```python
from build123d import *

# Parameters (mm, degrees)
ESQUISSE1_W                                        = 50.5
ESQUISSE1_H                                        = 26.5
ESQUISSE1_R                                        = 1.1
BOSS_EXTRU_1_DEPTH                                 = 3
CONG_1_R                                           = 1
CHAMBRAGE_POUR_VIS_SIX_PANS_CREUX_M1_6_D           = 2.2
CHAMBRAGE_POUR_VIS_SIX_PANS_CREUX_M1_6_CBORE_D     = 3.8
CHAMBRAGE_POUR_VIS_SIX_PANS_CREUX_M1_6_CBORE_DEPTH = 1.2
BOSS_EXTRU_2_START                                 = -19
ESQUISSE4_R                                        = 1.6
ESQUISSE4_W                                        = 11.6
ESQUISSE4_H                                        = 26.5
BOSS_EXTRU_2_DEPTH                                 = 19
ENL_V_START                                        = -19
ENL_V_MAT_EXTRU_1_DEPTH                            = 7
ESQUISSE6_W                                        = 11.6
ESQUISSE6_H                                        = 6
ENL_V_MAT_EXTRU_2_DEPTH                            = 50.487191272
BOSS_EXTRU_3_DEPTH                                 = 2
CHANFREIN1_SIZE                                    = 1


with BuildPart() as part:
    # Esquisse1 → Boss.-Extru.1 (new body)
    with BuildSketch(Plane(origin=(0, 0, 0), x_dir=(1, 0, 0), z_dir=(0, 1, 0))):
        with Locations((4.2, 10.25)):
            Rectangle(ESQUISSE1_W, ESQUISSE1_H)
        with Locations(Location((0, 0, 0), (0, 0, 270))):
            Circle(ESQUISSE1_R, mode=Mode.SUBTRACT)
        with Locations(Location((24.45, 0, 0), (0, 0, 270))):
            Circle(ESQUISSE1_R, mode=Mode.SUBTRACT)
        with BuildLine():
            Line((8.89, 20.95), (8.89, 19.74))
            Line((8.89, 19.74), (21.54, 19.74))
            Line((21.54, 19.74), (21.54, 0.76))
            Line((21.54, 0.76), (8.89, 0.76))
            Line((8.89, 0.76), (8.89, -0.45))
            Line((8.89, -0.45), (2.51, -0.45))
            Line((2.51, -0.45), (2.51, 6.385507795))
            ThreePointArc((2.51, 6.385507795), (-19.78, 10.25), (2.51, 14.114492205))
            Line((2.51, 14.114492205), (2.51, 20.95))
            Line((2.51, 20.95), (8.89, 20.95))
        make_face(mode=Mode.SUBTRACT)
        with Locations(Location((0, 20.5, 0), (0, 0, 270))):
            Circle(ESQUISSE1_R, mode=Mode.SUBTRACT)
        with Locations(Location((24.45, 20.5, 0), (0, 0, 270))):
            Circle(ESQUISSE1_R, mode=Mode.SUBTRACT)
    extrude(amount=BOSS_EXTRU_1_DEPTH)

    # Congé1
    cong_1_edges = [part.edges().sort_by_distance(p)[0] for p in [
        (2.51, 1.5, -6.385507795),
        (2.51, 1.5, -14.114492205),
    ]]
    fillet(cong_1_edges, radius=CONG_1_R)

    # Chambrage pour vis à six pans creux M1.61 (through all)
    with Locations(Plane(origin=(0, 3, 0), x_dir=(1, 0, 0), z_dir=(0, 1, 0))):
        with Locations((0, 0), (0, 20.5), (24.45, 20.5), (24.45, 0)):
            CounterBoreHole(CHAMBRAGE_POUR_VIS_SIX_PANS_CREUX_M1_6_D / 2, CHAMBRAGE_POUR_VIS_SIX_PANS_CREUX_M1_6_CBORE_D / 2, CHAMBRAGE_POUR_VIS_SIX_PANS_CREUX_M1_6_CBORE_DEPTH)

    # Esquisse4 → Boss.-Extru.2 (add)
    # profile 1 of 2: a face of its own
    with BuildSketch(Plane(origin=(0, 3, 0), x_dir=(1, 0, 0), z_dir=(0, 1, 0)).offset(BOSS_EXTRU_2_START)):
        with BuildLine():
            Line((-18.61, 23.5), (-30.21, 23.5))
            Line((-30.21, 23.5), (-30.21, -3))
            Line((-30.21, -3), (-18.61, -3))
            Line((-18.61, -3), (-18.61, 5.200811946))
            ThreePointArc((-18.61, 5.200811946), (-19.78, 10.25), (-18.61, 15.299188054))
            Line((-18.61, 15.299188054), (-18.61, 23.5))
        make_face()
        with Locations(Location((-24.41, 10.25, 0), (0, 0, 270))):
            Circle(ESQUISSE4_R, mode=Mode.SUBTRACT)
    # profile 2 of 2: a face of its own
    with BuildSketch(Plane(origin=(0, 3, 0), x_dir=(1, 0, 0), z_dir=(0, 1, 0)).offset(BOSS_EXTRU_2_START)):
        with Locations((32.81, 10.25)):
            Rectangle(ESQUISSE4_W, ESQUISSE4_H)
        with Locations(Location((32.81, 3, 0), (0, 0, 90))):
            Circle(ESQUISSE4_R, mode=Mode.SUBTRACT)
        with Locations(Location((32.81, 17.5, 0), (0, 0, 90))):
            Circle(ESQUISSE4_R, mode=Mode.SUBTRACT)
    extrude(amount=BOSS_EXTRU_2_DEPTH)

    # Esquisse5 → Enlèv. mat.-Extru.1 (cut)
    with BuildSketch(Plane.XZ.offset(16).offset(ENL_V_START)):
        Polygon((-24.41, -7.016838493), (-27.21, -8.633419246), (-27.21, -11.866580754), (-24.41, -13.483161507), (-21.61, -11.866580754), (-21.61, -8.633419246), align=None)
        Polygon((32.81, -14.266838493), (30.01, -15.883419246), (30.01, -19.116580754), (32.81, -20.733161507), (35.61, -19.116580754), (35.61, -15.883419246), align=None)
        Polygon((32.81, 0.233161507), (30.01, -1.383419246), (30.01, -4.616580754), (32.81, -6.233161507), (35.61, -4.616580754), (35.61, -1.383419246), align=None)
    extrude(amount=ENL_V_MAT_EXTRU_1_DEPTH, mode=Mode.SUBTRACT)

    # Esquisse6 → Enlèv. mat.-Extru.2 (cut, through all)
    with BuildSketch(Plane(origin=(0, 0, -23.5), x_dir=(-1, 0, 0), z_dir=(0, 0, -1))):
        with Locations((-32.81, -13)):
            Rectangle(ESQUISSE6_W, ESQUISSE6_H)
        with Locations((24.41, -13)):
            Rectangle(ESQUISSE6_W, ESQUISSE6_H)
    extrude(amount=-ENL_V_MAT_EXTRU_2_DEPTH, mode=Mode.SUBTRACT)

    # Esquisse7 → Boss.-Extru.3 (add)
    with BuildSketch(Plane(origin=(0, 0, -23.5), x_dir=(-1, 0, 0), z_dir=(0, 0, -1))):
        Polygon((8.61, 0), (-4.2, 0), (-17.01, 0), (-22.01, -5), (13.61, -5), align=None)
        Polygon((-22.01, -5), (-17.01, 0), (-27.01, 0), (-27.01, -10), align=None)
        Polygon((-17.01, 0), (-4.2, 0), (-4.2, 3), (-38.61, 3), (-38.61, -10), (-27.01, -10), (-27.01, 0), align=None)
        Polygon((18.61, 0), (8.61, 0), (13.61, -5), (18.61, -10), align=None)
        Polygon((-4.2, 3), (-4.2, 0), (8.61, 0), (18.61, 0), (18.61, -10), (30.21, -10), (30.21, 3), align=None)
    boss_extru_3 = extrude(amount=BOSS_EXTRU_3_DEPTH)

    # Symétrie1: Boss.-Extru.3 across plane
    add(boss_extru_3.mirror(Plane(origin=(0, 0, -10.25), x_dir=(1, 0, 0), z_dir=(0, 0, -1))))

    # Chanfrein1
    chanfrein1_edges = [part.edges().sort_by_distance(p)[0] for p in [
        (-30.21, 3, -10.25),
        (38.61, 3, -10.25),
        (-30.21, -3.5, -25.5),
        (4.2, 3, -25.5),
        (38.61, -3.5, -25.5),
        (38.61, -3.5, 5),
        (4.2, 3, 5),
        (-30.21, -3.5, 5),
    ]]
    chamfer(chanfrein1_edges, length=CHANFREIN1_SIZE)


solid = part.part
```
Verification items for the finished model (mm, model axes). A direction names the side the tool comes from. Round coordinates to 2 decimals unless told otherwise and drop trailing zeros. Order: outer loops, then holes, each group sorted by start corner. A loop starts at its lowest first (then second) coordinate and runs counter-clockwise, first axis right, second up. Notation, with made-up numbers: (-22.5, 27.5) - (5.5, 27.5) arc R18 ccw to (5.5, 33.5) - close; hole circle Ø3 at (35, -15.5). An arc over 180 degrees is marked (long way). Use CSV: the item, a comma, the result in double quotes. Start each with the question number.
1) Go/stop test with flat-tipped pins: P1, Ø1.3, axis at x = 0, z = 0, coming from the -Y side; P2, Ø1.1, axis at x = 0.5, z = -21, coming from the +Y side. Record where each tip stops, or that it passes through.
2) Thickness scan on L1, parallel to X at y = -8.05, z = -17.5; L2, parallel to X at y = -1, z = -18.5; L3, parallel to Z at x = 24.45, y = 1.1. Record the ranges inside material, lowest first.
3) Mould release check, pull along Z, two halves, no side actions. Record for faces 1 (the cylindrical face through (23.78, 0.89, -21.37)), 2 (the flat face through (-30.21, -4, -10)): +Z half, -Z half, draft (parallel to the pull), parting line (faces both ways), or undercut.
4) Section check B-B, the plane x = 20. Record the cut outline in (y, z).
5) Access from +Z, -Z, +X, -X, +Y, -Y to the whole of each face (thin tool, end or side, straight path). Record for faces 3 (the flat face through (-22.99, -0.451, -7.836)), 4 (the flat face through (5, -3, 3)), 5 (the flat face through (2.51, 1, -19)).
6) Section check C-C, the plane y = -3. State how many separate pieces and enclosed holes the cut face has, plus the area to 3 significant figures.
7) Section check D-D, the plane z = -10.25. Record the cut outline in (x, y), plus the area to 3 significant figures.
8) Section check A-A, the plane y = -7.5. Record the cut outline in (x, z).
Answers:
1,P1,"passes through"
1,P2,"stops at y = 1.8"
2,L1,"x = -30.21 to -18.61, 27.01 to 31.21, 34.41 to 38.61"
2,L2,"x = -30.21 to -18.61, 27.01 to 30.01, 35.61 to 38.61"
2,L3,"z = -25.5 to -21.6, -19.4 to -1.1, 1.1 to 5"
3,face 1,"undercut"
3,face 2,"draft"
4,outline,"(-5, -25.5) - (2, -25.5) - (3, -24.5) - (3, -19.74) - (0, -19.74) - (0, -23.5) - (-5, -23.5) - close; (-5, 3) - (0, 3) - (0, -0.76) - (3, -0.76) - (3, 4) - (2, 5) - (-5, 5) - close"
5,face 3,"+Y"
5,face 4,"-Y"
5,face 5,"+Y, -Y"
6,separate pieces,"1"
6,enclosed holes,"4"
6,area,"799 mm²"
7,outline,"(-30.21, -10) - (-26.01, -10) - (-26.01, -4) - (-27.21, -4) - (-27.21, 3) - (-29.21, 3) - (-30.21, 2) - close; (-22.81, -10) - (-19.78, -10) - (-19.78, 3) - (-21.61, 3) - (-21.61, -4) - (-22.81, -4) - close; (21.54, 0) - (27.01, 0) - (27.01, -10) - (38.61, -10) - (38.61, 2) - (37.61, 3) - (21.54, 3) - close"
7,area,"243 mm²"
8,outline,"(-30.21, -24.5) - (-29.21, -25.5) - (-16.11, -25.5) - (-16.11, -23.5) - (-18.61, -23.5) - (-18.61, -15.3) arc R11.48 cw to (-18.61, -5.2) - (-18.61, 3) - (-16.11, 3) - (-16.11, 5) - (-29.21, 5) - (-30.21, 4) - close; (24.51, -25.5) - (37.61, -25.5) - (38.61, -24.5) - (38.61, 4) - (37.61, 5) - (24.51, 5) - (24.51, 3) - (27.01, 3) - (27.01, -23.5) - (24.51, -23.5) - close; hole circle Ø3.2 at (-24.41, -10.25); hole circle Ø3.2 at (32.81, -17.5); hole circle Ø3.2 at (32.81, -3)"
